Autodesk Inventor part; units mm, degrees
ref_plane "YZ Plane" through (0, 0, 0) normal (1, 0, 0) x (0, 1, 0)
ref_plane "XZ Plane" through (0, 0, 0) normal (0, 1, 0) x (-1, 0, 0)
ref_plane "XY Plane" through (0, 0, 0) normal (0, 0, 1) x (1, 0, 0)
sketch "Sketch2" plane through (0, 0, 1) normal (0, 0, 1) x (1, 0, 0)
  line L0 (-17.5, 32.5) -> (-12.5, 32.5)
  line L1 (-7.5, 27.5) -> (-7.5, 12.5)
  line L2 (-12.5, 7.5) -> (-17.5, 7.5)
  line L3 (-22.5, 12.5) -> (-22.5, 27.5)
  line L4 (-22.5, 32.5) -> (-7.5, 7.5) construction
  line L5 (-7.5, 32.5) -> (-22.5, 7.5) construction
  line L6 (-15.4861, 0) -> (17.9861, 0)
  line L7 (0, 18.4722) -> (0, -18.4722)
  arc A0 (-17.5, 32.5) -> (-22.5, 27.5) centre (-17.5, 27.5) ccw
  arc A1 (-7.5, 27.5) -> (-12.5, 32.5) centre (-12.5, 27.5) ccw
  arc A2 (-12.5, 7.5) -> (-7.5, 12.5) centre (-12.5, 12.5) ccw
  arc A3 (-22.5, 12.5) -> (-17.5, 7.5) centre (-17.5, 12.5) ccw
  line L8 (17.5, 32.5) -> (12.5, 32.5)
  line L9 (7.5, 27.5) -> (7.5, 12.5)
  line L10 (12.5, 7.5) -> (17.5, 7.5)
  line L11 (22.5, 12.5) -> (22.5, 27.5)
  line L12 (22.5, 32.5) -> (7.5, 7.5) construction
  line L13 (7.5, 32.5) -> (22.5, 7.5) construction
  arc A4 (22.5, 27.5) -> (17.5, 32.5) centre (17.5, 27.5) ccw
  arc A5 (12.5, 32.5) -> (7.5, 27.5) centre (12.5, 27.5) ccw
  arc A6 (7.5, 12.5) -> (12.5, 7.5) centre (12.5, 12.5) ccw
  arc A7 (17.5, 7.5) -> (22.5, 12.5) centre (17.5, 12.5) ccw
  line L14 (-17.5, -32.5) -> (-12.5, -32.5)
  line L15 (-7.5, -27.5) -> (-7.5, -12.5)
  line L16 (-12.5, -7.5) -> (-17.5, -7.5)
  line L17 (-22.5, -12.5) -> (-22.5, -27.5)
  line L18 (-22.5, -32.5) -> (-7.5, -7.5) construction
  line L19 (-7.5, -32.5) -> (-22.5, -7.5) construction
  arc A8 (-22.5, -27.5) -> (-17.5, -32.5) centre (-17.5, -27.5) ccw
  arc A9 (-12.5, -32.5) -> (-7.5, -27.5) centre (-12.5, -27.5) ccw
  arc A10 (-7.5, -12.5) -> (-12.5, -7.5) centre (-12.5, -12.5) ccw
  arc A11 (-17.5, -7.5) -> (-22.5, -12.5) centre (-17.5, -12.5) ccw
  line L20 (12.5, -7.5) -> (17.5, -7.5)
  line L21 (7.5, -27.5) -> (7.5, -12.5)
  arc A12 (22.5, -12.5) -> (17.5, -7.5) centre (17.5, -12.5) ccw
  arc A13 (7.5, -27.5) -> (12.5, -32.5) centre (12.5, -27.5) ccw
  line L22 (17.5, -32.5) -> (12.5, -32.5)
  line L23 (7.5, -32.5) -> (22.5, -7.5) construction
  line L24 (22.5, -32.5) -> (7.5, -7.5) construction
  line L25 (22.5, -12.5) -> (22.5, -27.5)
  arc A14 (17.5, -32.5) -> (22.5, -27.5) centre (17.5, -27.5) ccw
  arc A15 (12.5, -7.5) -> (7.5, -12.5) centre (12.5, -12.5) ccw
  point P0 (0, 0)
  point P1 (-15, 20)
  point P2 (15, 20)
  point P3 (-15, -20)
  point P4 (15, -20)
  dimension "d11" = 15
  dimension "d12" = 15
  dimension "d13" = 25
  dimension "d14" = 15
  dimension "d15" = 5
sketch "Sketch1" plane through (0, 0, 0) normal (0, 0, 1) x (1, 0, 0)
  line L0 (-36, 10) -> (36, 10)
  line L1 (36, 10) -> (36, -10)
  line L2 (36, -10) -> (-36, -10)
  line L3 (-36, -10) -> (-36, 10)
  line L4 (-36, 10) -> (36, -10) construction
  line L5 (36, 10) -> (-36, -10) construction
  circle A0 centre (31.1, 0) radius 1.6
  line L6 (0, 0) -> (12.8976, 0)
  line L7 (0, 0) -> (0, 11.3109)
  circle A1 centre (-31.1, 0) radius 1.6
  circle A2 centre (0, -4) radius 1.6
  circle A3 centre (0, 4) radius 1.6
  dimension "d0" = 72
  dimension "d1" = 20
  dimension "d2" = 3.2
  dimension "d3" = 4.9
  dimension "d6" = 3.2
  dimension "d7" = 6
extrude "Plate1" add sketch "Sketch1" along normal blind 1
sketch "Sketch3" plane through (0, 0, 1) normal (0, 0, 1) x (1, 0, 0)
  line L0 (-16, 5) -> (-14, 5)
  line L1 (-10, 1) -> (-10, -1)
  line L2 (-14, -5) -> (-16, -5)
  line L3 (-20, -1) -> (-20, 1)
  line L4 (-20, 5) -> (-10, -5) construction
  line L5 (-10, 5) -> (-20, -5) construction
  arc A0 (-16, 5) -> (-20, 1) centre (-16, 1) ccw
  arc A1 (-20, -1) -> (-16, -5) centre (-16, -1) ccw
  arc A2 (-14, -5) -> (-10, -1) centre (-14, -1) ccw
  arc A3 (-10, 1) -> (-14, 5) centre (-14, 1) ccw
  line L6 (0, 0) -> (0, 13.3665)
  line L7 (16, 5) -> (14, 5)
  line L8 (10, 1) -> (10, -1)
  line L9 (14, -5) -> (16, -5)
  line L10 (20, -1) -> (20, 1)
  line L11 (20, 5) -> (10, -5) construction
  line L12 (10, 5) -> (20, -5) construction
  arc A4 (20, 1) -> (16, 5) centre (16, 1) ccw
  arc A5 (16, -5) -> (20, -1) centre (16, -1) ccw
  arc A6 (10, -1) -> (14, -5) centre (14, -1) ccw
  arc A7 (14, 5) -> (10, 1) centre (14, 1) ccw
  point P0 (-15, 0)
  point P1 (15, 0)
  dimension "d18" = 10
  dimension "d19" = 10
  dimension "d20" = 4
  dimension "d21" = 20
extrude "Cut2" cut sketch "Sketch3" against normal blind 1
equation "\"d22\" = 厚度"
equation "\"d5\" = 厚度"
equation "\"折彎半徑\" = 厚度"
equation "\"折彎離隙寬度\" = 厚度"
equation "\"折彎離隙深度\" = 0.5 * 厚度"
equation "\"轉角離隙大小\" = 4 * 厚度"
equation "\"最小剩餘\" = 2 * 厚度"
equation "\"轉移半徑\" = 折彎半徑"
equation "\"Jacobi半徑大小\" = 折彎半徑"
equation "\"間隙大小\" = 厚度"
properties part number "battery_box_5V_front" material "Aluminum"
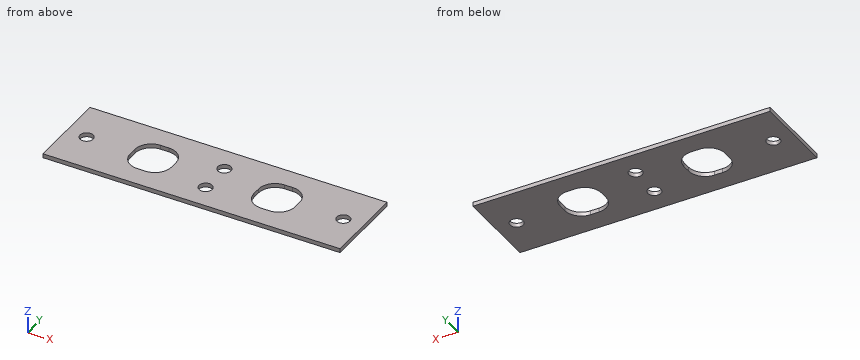
Part model, mm, in its own coordinate system. Give positions to 0.01 mm unless a question says otherwise; leave off trailing zeros. Order: outer loops, then holes, each group sorted by start corner. A loop starts at its lowest first (then second) coordinate and runs counter-clockwise, first axis right, second up. Notation, with made-up numbers: (-12.75, 66) - (44.25, 66) arc R27 ccw to (44.25, 100) - close; hole circle Ø3 at (85.5, -25). An arc over 180 degrees is marked (long way). One line per question, with ' | ' between items.
1. Drill centre lines: probe 1 along Y at (x, z) = (0, 0.5); probe 2 along X at (y, z) = (-0.75, 0.8); probe 3 along X at (y, z) = (-2, 0.85). Where is each one in solid material? Low to high.
Filled in:
probe 1: -10 to -5.6, -2.4 to 2.4, 5.6 to 10 | probe 2: -36 to -32.51, -29.69 to -20, -10 to 10, 20 to 29.69, 32.51 to 36 | probe 3: -36 to -19.87, -10.13 to 10.13, 19.87 to 36
2. Drop a flat-ended pin along its axis: P1, Ø2.5, axis at x = 0, y = 4, coming from the +Z side. Give the stop position or say it passes through.
Filled in:
P1: through
3. Band-saw the part on C-C on x = -31.1. List the corners of the cut face in (y, z), then the cut area to 3 significant figures.
Filled in:
outline: (-10, 0) - (-1.6, 0) - (-1.6, 1) - (-10, 1) - close; (1.6, 0) - (10, 0) - (10, 1) - (1.6, 1) - close | area: 16.8 mm²
4. Band-saw the part on B-B on y = -4. List the corners of the cut face in (x, z).
Filled in:
outline: (-36, 0) - (-18.65, 0) - (-18.65, 1) - (-36, 1) - close; (-11.35, 0) - (-1.6, 0) - (-1.6, 1) - (-11.35, 1) - close; (1.6, 0) - (11.35, 0) - (11.35, 1) - (1.6, 1) - close; (18.65, 0) - (36, 0) - (36, 1) - (18.65, 1) - close
5. Band-saw the part on A-A on x = 0. List the corners of the cut face in (y, z).
Filled in:
outline: (-10, 0) - (-5.6, 0) - (-5.6, 1) - (-10, 1) - close; (-2.4, 0) - (2.4, 0) - (2.4, 1) - (-2.4, 1) - close; (5.6, 0) - (10, 0) - (10, 1) - (5.6, 1) - close
6. Band-saw the part on D-D on z = 0.5. List the corners of the cut face in (x, y).
Filled in:
outline: (-36, -10) - (36, -10) - (36, 10) - (-36, 10) - close; hole circle Ø3.2 at (-31.1, 0); hole (-20, -1) arc R4 ccw to (-16, -5) - (-14, -5) arc R4 ccw to (-10, -1) - (-10, 1) arc R4 ccw to (-14, 5) - (-16, 5) arc R4 ccw to (-20, 1) - close; hole circle Ø3.2 at (0, -4); hole circle Ø3.2 at (0, 4); hole (10, -1) arc R4 ccw to (14, -5) - (16, -5) arc R4 ccw to (20, -1) - (20, 1) arc R4 ccw to (16, 5) - (14, 5) arc R4 ccw to (10, 1) - close; hole circle Ø3.2 at (31.1, 0)
